Geometry check sheet. Reference: the model listing, model coordinates, mm. Round coordinates to 2 decimals unless told otherwise and drop trailing zeros. Loops run counter-clockwise (first coordinate to the right, second up) from the corner with the lowest first, then second, coordinate; pieces in that order, holes last. Notation, with made-up numbers: (22, 35) - (34, 35) arc R24 cw to (34, 58) - close; hole circle Ø1 at (31, -10). An arc over 180 degrees is marked (long way). Answer as CSV lines item,"result". Start each with the question number.
1) Thickness scan on line 1 along X through (y, z) = (3.5, -60); line 2 along X through (y, z) = (3.55, 10); line 3 along Z through (x, y) = (10.5, 2.25). Record the ranges inside material, lowest first.
2) Cross-section at A-A on z = 40. Record the boundary of the cut face in (x, y).
3) Cross-section at D-D on x = 79.5. Record the boundary of the cut face in (y, z).
4) Depth check by flat-ended pin: P1, Ø6, axis at x = 88.5, z = -60, coming from the -Y side. Enter the tip coordinate at first touch or a pass-through.
5) Cross-section at B-B on x = 14. Record the boundary of the cut face in (y, z), and give its area (3 significant figures).
6) Cross-section at C-C on y = 1.35. Record the boundary of the cut face in (x, z) (3 decimals).
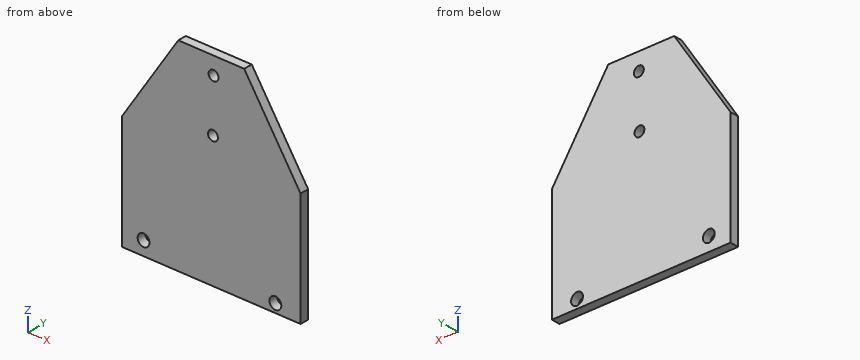
from build123d import *

# Parameters (mm, degrees)
SKETCH1_R               = 3.415098232
SKETCH1_R_2             = 3.415
BOSS_EXTRUDE1_DEPTH     = 5
CUT_EXTRUDE1_DEPTH      = 122.897497923
CUT_EXTRUDE1_DEPTH_BACK = 122.897497923
SKETCH2_R               = 2.85


with BuildPart() as part:
    # Sketch1 → Boss-Extrude1 (new body)
    with BuildSketch(Plane(origin=(0, 0, 0), x_dir=(1, 0, 0), z_dir=(0, 1, 0))):
        Polygon((0, 0), (0, 65), (103, 65), (103, 0), (70.5, -50), (32.5, -50), align=None)
        with Locations(Location((88.5, 60, 0), (0, 0, 270))):
            Circle(SKETCH1_R, mode=Mode.SUBTRACT)
        with Locations(Location((12.5, 57, 0), (0, 0, 270))):
            Circle(SKETCH1_R_2, mode=Mode.SUBTRACT)
    extrude(amount=BOSS_EXTRUDE1_DEPTH)

    # Sketch2 → Cut-Extrude1 (cut, two sides: drawn at the far end of the back side and taken through both)
    with BuildSketch(Plane(origin=(0, 5, 0), x_dir=(1, 0, 0), z_dir=(0, 1, 0)).offset(-CUT_EXTRUDE1_DEPTH_BACK)):
        with Locations(Location((52.841163777, -40, 0), (0, 0, 270))):
            Circle(SKETCH2_R)
        with Locations(Location((52.511369406, -10, 0), (0, 0, 270))):
            Circle(SKETCH2_R)
    extrude(amount=CUT_EXTRUDE1_DEPTH + CUT_EXTRUDE1_DEPTH_BACK, mode=Mode.SUBTRACT)


solid = part.part
Answer block:
1,line 1,"x = 0 to 10.87, 14.13 to 85.08, 91.92 to 103"
1,line 2,"x = 6.5 to 49.66, 55.36 to 96.5"
1,line 3,"z = -65 to -59.77, -54.23 to 16.15"
2,outline,"(26, 0) - (49.99, 0) - (49.99, 5) - (26, 5) - close; (55.69, 0) - (77, 0) - (77, 5) - (55.69, 5) - close"
3,outline,"(0, -65) - (5, -65) - (5, 36.15) - (0, 36.15) - close"
4,P1,"passes through"
5,outline,"(0, -65) - (5, -65) - (5, -60.07) - (0, -60.07) - close; (0, -53.93) - (5, -53.93) - (5, 21.54) - (0, 21.54) - close"
5,area,"402 mm^2"
6,outline,"(0, -65) - (103, -65) - (103, 0) - (70.5, 50) - (32.5, 50) - (0, 0) - close; hole circle Ø6.83 at (12.5, -57); hole circle Ø5.7 at (52.511, 10); hole circle Ø5.7 at (52.841, 40); hole circle Ø6.83 at (88.5, -60)"
